Verification items for the finished model (mm, model axes). Coordinates: 2 decimals unless noted, no trailing zeros. Order: outer loops, then holes, each group sorted by start corner. A loop starts at its lowest first (then second) coordinate and runs counter-clockwise, first axis right, second up. Notation, with made-up numbers: (36.5, -31.75) -> (92.5, -31.75) arc R25 ccw to (92.5, 4.25) -> close; hole circle Ø5 at (46, 1.25). An arc over 180 degrees is marked (long way). Write item = value, one per line. Start each with the question number.
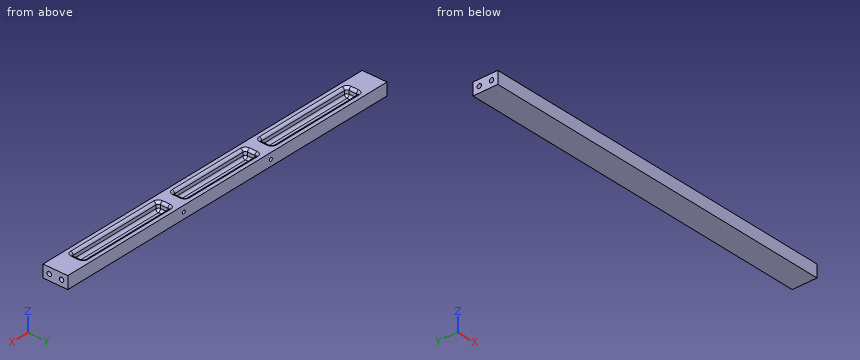
from build123d import *

# Parameters (mm, degrees)
SKETCH1_W                  = 558.8
SKETCH1_H                  = 38.1
EXTRUDE1_DEPTH             = 9.525
M8X1_25_TAPPED_HOLE1_D     = 6.8
M8X1_25_TAPPED_HOLE1_DEPTH = 19.812
M8X1_25_TAPPED_HOLE1_TIP   = 2.042926105
M8X1_25_TAPPED_HOLE2_D     = 6.8
M8X1_25_TAPPED_HOLE2_DEPTH = 19.812
M8X1_25_TAPPED_HOLE2_TIP   = 2.042926105
M6X1_0_TAPPED_HOLE1_D      = 5
M6X1_0_TAPPED_HOLE1_DEPTH  = 12.7
M6X1_0_TAPPED_HOLE1_TIP    = 1.502151548
SKETCH12_W                 = 127
SKETCH12_H                 = 19.05
SKETCH12_W_2               = 152.4
CUT_EXTRUDE1_DEPTH         = 12.7
FILLET1_R                  = 3.81


with BuildPart() as part:
    # Sketch1 → Extrude1 (new body, symmetric)
    with BuildSketch(Plane.XY):
        Rectangle(SKETCH1_W, SKETCH1_H)
    extrude(amount=EXTRUDE1_DEPTH, both=True)

    # M8x1.25 Tapped Hole1
    with Locations(Plane.ZY.offset(279.4)):
        with Locations((0, 9.525), (0, -9.525)):
            Hole(M8X1_25_TAPPED_HOLE1_D / 2, depth=M8X1_25_TAPPED_HOLE1_DEPTH)
            with Locations((0, 0, -(M8X1_25_TAPPED_HOLE1_DEPTH + M8X1_25_TAPPED_HOLE1_TIP / 2))):  # 118° drill point
                Cone(0, M8X1_25_TAPPED_HOLE1_D / 2, M8X1_25_TAPPED_HOLE1_TIP, mode=Mode.SUBTRACT)

    # M8x1.25 Tapped Hole2
    with Locations(Plane(origin=(279.4, 0, 0), x_dir=(0, 0, -1), z_dir=(1, 0, 0))):
        with Locations((0, 9.525), (0, -9.525)):
            Hole(M8X1_25_TAPPED_HOLE2_D / 2, depth=M8X1_25_TAPPED_HOLE2_DEPTH)
            with Locations((0, 0, -(M8X1_25_TAPPED_HOLE2_DEPTH + M8X1_25_TAPPED_HOLE2_TIP / 2))):  # 118° drill point
                Cone(0, M8X1_25_TAPPED_HOLE2_D / 2, M8X1_25_TAPPED_HOLE2_TIP, mode=Mode.SUBTRACT)

    # M6x1.0 Tapped Hole1
    with Locations(Plane(origin=(0, 19.05, 0), x_dir=(1, 0, 0), z_dir=(0, 1, 0))):
        with Locations((-76.2, 0), (76.2, 0)):
            Hole(M6X1_0_TAPPED_HOLE1_D / 2, depth=M6X1_0_TAPPED_HOLE1_DEPTH)
            with Locations((0, 0, -(M6X1_0_TAPPED_HOLE1_DEPTH + M6X1_0_TAPPED_HOLE1_TIP / 2))):  # 118° drill point
                Cone(0, M6X1_0_TAPPED_HOLE1_D / 2, M6X1_0_TAPPED_HOLE1_TIP, mode=Mode.SUBTRACT)

    # Sketch12 → Cut-Extrude1 (cut)
    with BuildSketch(Plane.XY.offset(9.525)):
        Rectangle(SKETCH12_W, SKETCH12_H)
        with Locations((165.1, 0)):
            Rectangle(SKETCH12_W_2, SKETCH12_H)
        with Locations((-165.1, 0)):
            Rectangle(SKETCH12_W_2, SKETCH12_H)
    extrude(amount=-CUT_EXTRUDE1_DEPTH, mode=Mode.SUBTRACT)

    # Fillet1
    fillet1_edges = [part.edges().sort_by_distance(p)[0] for p in [
        (-88.9, 0, -3.175),
        (-88.9, 9.525, 3.175),
        (-165.1, -9.525, -3.175),
        (-88.9, -9.525, 3.175),
        (-241.3, 0, -3.175),
        (-241.3, -9.525, 3.175),
        (-165.1, 9.525, -3.175),
        (-241.3, 9.525, 3.175),
        (-88.9, 0, 9.525),
        (-165.1, 9.525, 9.525),
        (-241.3, 0, 9.525),
        (-165.1, -9.525, 9.525),
        (241.3, 9.525, 3.175),
        (165.1, -9.525, -3.175),
        (241.3, -9.525, 3.175),
        (88.9, 0, -3.175),
        (88.9, -9.525, 3.175),
        (165.1, 9.525, -3.175),
        (88.9, 9.525, 3.175),
        (241.3, 0, 9.525),
        (165.1, 9.525, 9.525),
        (88.9, 0, 9.525),
        (165.1, -9.525, 9.525),
        (63.5, 0, -3.175),
        (63.5, 9.525, 3.175),
        (0, -9.525, -3.175),
        (63.5, -9.525, 3.175),
        (-63.5, 0, -3.175),
        (-63.5, -9.525, 3.175),
        (0, 9.525, -3.175),
        (-63.5, 9.525, 3.175),
        (63.5, 0, 9.525),
        (0, 9.525, 9.525),
        (-63.5, 0, 9.525),
        (0, -9.525, 9.525),
    ]]
    fillet(fillet1_edges, radius=FILLET1_R)


solid = part.part
Item 1: Gauge pin test, flat ends, axial feed: P1, Ø4, axis at y = 9.525, z = 0, coming from the -X side; P2, Ø10, axis at x = 34.5, y = -0.5, coming from the +Z side (3 decimals); P3, Ø6, axis at y = 9.525, z = 0, coming from the -X side. Record the tip position at first contact, or that the pin passes through.
Item 2: Section check A-A (x = 137). Record the boundary of the cut face in (y, z) (3 decimals), then the cut area to 3 significant figures.
Item 3: Thickness scan on line 1 (Y direction, x = 270.5, z = 0) (3 decimals); line 2 (Y direction, x = -232.5, z = 3.5) (3 decimals); line 3 (X direction, y = 16.5, z = -0.75). Record the ranges inside material, lowest first.
Filled sheet:
q1.P1 = -258.75
q1.P2 = -3.175
q1.P3 = -259.35
q2.outline = (-19.05, -9.525) -> (19.05, -9.525) -> (19.05, 9.525) -> (13.335, 9.525) arc R3.81 ccw to (9.525, 5.715) -> (9.525, 0.635) arc R3.81 cw to (5.715, -3.175) -> (-5.715, -3.175) arc R3.81 cw to (-9.525, 0.635) -> (-9.525, 5.715) arc R3.81 ccw to (-13.335, 9.525) -> (-19.05, 9.525) -> close
q2.area = 484 mm^2
q3.line_1 = -19.05 to -12.925, -6.125 to 6.125, 12.925 to 19.05
q3.line_2 = -19.05 to -9.525, 9.525 to 19.05
q3.line_3 = -279.4 to -78.58, -73.82 to 73.82, 78.58 to 279.4
